Autodesk Inventor part; units mm, degrees
ref_plane "YZ Plane" through (0, 0, 0) normal (1, 0, 0) x (0, 1, 0)
ref_plane "XZ Plane" through (0, 0, 0) normal (0, 1, 0) x (-1, 0, 0)
ref_plane "XY Plane" through (0, 0, 0) normal (0, 0, 1) x (1, 0, 0)
sketch "草圖1" plane through (0, 0, 0) normal (0, 1, 0) x (-1, 0, 0)
  line L0 (0, 0) -> (-70, 0)
  line L1 (-70, 0) -> (-70, 40)
  line L2 (-70, 40) -> (0, 40)
  line L3 (0, 40) -> (0, 0)
  dimension "d0" = 70
  dimension "d1" = 40
extrude "擠出1" add sketch "草圖1" along normal blind 10
sketch "草圖2" plane through (0, 10, 0) normal (0, 1, 0) x (1, 0, 0)
  line L0 (0, -40) -> (0, 0)
  line L1 (0, 0) -> (70, 0)
  line L2 (70, 0) -> (70, -40)
  line L3 (70, -40) -> (0, -40)
  line L4 (0, 0) -> (70, 0)
  line L5 (70, 0) -> (70, -20)
  line L6 (70, -20) -> (0, -20)
  line L7 (0, -20) -> (0, 0)
  line L8 (70, -40) -> (70, 0)
  line L9 (40, -20) -> (50, -10)
  line L10 (50, -10) -> (70, -10)
  point P0 (0, -20)
  dimension "d4" = 20
  dimension "d5" = 10
  dimension "d6" = 20
  dimension "d7" = 30
extrude "擠出2" add sketch "草圖2" along normal blind 30 contours L0 L1 L2 L10 L9 L6
sketch "草圖3" plane through (50, 10, 10) normal (0, 0, 1) x (1, 0, 0)
  line L0 (0, 30) -> (0, 0)
  line L1 (0, 0) -> (20, 0)
  line L2 (20, 0) -> (20, -10)
  line L3 (20, -10) -> (-50, -10)
  line L4 (-50, -10) -> (-50, 30)
  line L5 (-50, 30) -> (0, 30)
  line L6 (0, 30) -> (20, 30)
  line L7 (20, 30) -> (20, 0)
  line L8 (0, 30) -> (20, 30)
  line L9 (20, 0) -> (0, 0)
  line L10 (0, 30) -> (20, 0)
extrude "擠出3" cut sketch "草圖3" against normal blind 10 contours L6 L7 L10
sketch "草圖4" plane through (0, 10, 20) normal (0, 0, 1) x (1, 0, 0)
  line L0 (0, -10) -> (0, 0)
  line L1 (0, 0) -> (0, 30)
  line L2 (0, 30) -> (40, 30)
  line L3 (40, 30) -> (40, 0)
  line L4 (40, 0) -> (70, 0)
  line L5 (70, 0) -> (70, -10)
  line L6 (70, -10) -> (0, -10)
  line L7 (0, 0) -> (40, 0)
  line L8 (0, 30) -> (40, 30)
  circle A0 centre (20, 30) radius 10
  dimension "d12" = 20
extrude "擠出4" cut sketch "草圖4" against normal blind 46 contours A0 L2 | L2 A0
properties part number "28" material "鋼、碳鋼"
For this review, take the finished solid that the model builds, in its own axes (mm). A direction names the side the tool comes from. Give positions to 0.01 mm unless a question says otherwise; leave off trailing zeros. Write each loop counter-clockwise with the first axis right and the second up, starting at its lowest first coordinate (ties: lowest second). Pieces come first, ordered by that corner, then holes. Notation, with made-up numbers: M 53,33.5 L 87,33.5 A30 cw 87,66.5 Z; hole C -28.75,26.5 d2. An arc over 180 degrees is marked long. One line per item, written item: value.
1) Take a section at B-B, the plane x = 20. Write out the cut boundary in (y, z).
Results are:
outline: M 0,0 L 30,0 L 30,20 L 10,20 L 10,40 L 0,40 Z
2) For faces 5 (the flat face through (5, 40, 10)), 6 (the flat face through (20, 21, 20)), 7 (the flat face through (35, 10, 29)), list the 3-axis set-ups (+Z, -Z, +X, -X, +Y, -Y) from which the entire face can be reached by the end or side of a thin tool; tool diameter is ignored.
Results are:
face 5: +Z, -Z, +X, -X, +Y
face 6: +Z, +X, -X, +Y
face 7: +Z, +X, +Y
3) For line 1 (Y direction, x = 42.5, z = 21); line 2 (Z direction, x = 34, y = 33); line 3 (X direction, y = 31.5, z = 6.5), list the stretches that pass through material, from the lowest coordinate up. Write a range as from..to.
Results are:
line 1: y = 0..10
line 2: z = 0..20
line 3: x = 0..14.73, 25.27..55.67
4) Take a section at C-C, the plane z = 19. Write out the cut boundary in (x, y).
Results are:
outline: M 0,0 L 70,0 L 70,10 L 41,10 L 41,40 L 30,40 A10 cw 10,40 L 0,40 Z
5) Take a section at D-D, the plane x = 48. Write out the cut boundary in (y, z), then the cut area to 3 significant figures.
Results are:
outline: M 0,0 L 40,0 L 40,12 L 10,12 L 10,40 L 0,40 Z
area: 760 mm²
6) The part is to be moulded in two halves that separate along X. For faces 1 (the cylindrical face through (20, 30, 10)), 2 (the flat face through (60, 25, 5)), 3 (the flat face through (35, 0, 20)), 4 (the flat face through (0, 15, 11)), say which applies: +X half, -X half, draft (parallel to the pull), parting line (faces both ways), or undercut.
Results are:
face 1: undercut
face 2: +X half
face 3: draft
face 4: -X half
7) For P1, Ø15, axis at x = 22.5, y = 31, coming from the +Z side; P2, Ø6, axis at x = 65, y = 18.5, coming from the +Z side; P3, Ø2, axis at x = 17, y = 32.5, coming from the +Z side, all flat-tipped, find the tip position at first contact; note any pin that passes through.
Results are:
P1: stops at z = 20
P2: stops at z = 10
P3: passes through
8) Take a section at A-A, the plane z = 12. Write out the cut boundary in (x, y).
Results are:
outline: M 0,0 L 70,0 L 70,10 L 48,10 L 48,40 L 30,40 A10 cw 10,40 L 0,40 Z
